Geometry check sheet. Reference: the model listing, model coordinates, mm. Round coordinates to 2 decimals unless told otherwise and drop trailing zeros. Order: outer loops, then holes, each group sorted by start corner. A loop starts at its lowest first (then second) coordinate and runs counter-clockwise, first axis right, second up.
(1) Cross-section at C-C on y = 1.75. Enter the section's corners in (x, z).
(2) Thickness scan on L1, parallel to X at y = 6.75, z = -0.25; L2, parallel to Z at x = -180, y = 6.25; L3, parallel to X at y = 6.5, z = -1. Record the ranges inside material, lowest first.
(3) Cross-section at A-A on z = 0. Enter the section's corners in (x, y).
(4) Gauge pin test, flat end, axial feed: P1, Ø1.5, axis at y = 3, z = -5.5, coming from the +X side. Record the tip position at first contact, or that the pin passes through.
(5) Cross-section at B-B on x = -160. Enter the section's corners in (y, z).
from build123d import *

# Parameters (mm, degrees)
BOSS_EXTRUDE1_DEPTH = 7.5
SKETCH2_R           = 2
CUT_EXTRUDE1_DEPTH  = 191.360841561
SKETCH3_R           = 5
CUT_EXTRUDE2_DEPTH  = 191.360841561


with BuildPart() as part:
    # Sketch1 → Boss-Extrude1 (new body)
    with BuildSketch(Plane(origin=(0, 0, 0), x_dir=(1, 0, 0), z_dir=(0, 1, 0))):
        with BuildLine():
            Line((0, 9), (-190, 9))
            Line((-190, 9), (-190, -9))
            Line((-190, -9), (0, -9))
            ThreePointArc((0, -9), (9, 0), (0, 9))
        make_face()
    extrude(amount=BOSS_EXTRUDE1_DEPTH)

    # Sketch2 → Cut-Extrude1 (cut, through all)
    with BuildSketch(Plane(origin=(0, 7.5, 0), x_dir=(1, 0, 0), z_dir=(0, 1, 0))):
        with Locations(Location((-180, 0, 0), (0, 0, 270))):
            Circle(SKETCH2_R)
        with Locations(Location((-160, 0, 0), (0, 0, 270))):
            Circle(SKETCH2_R)
    extrude(amount=-CUT_EXTRUDE1_DEPTH, mode=Mode.SUBTRACT)

    # Sketch3 → Cut-Extrude2 (cut, through all)
    with BuildSketch(Plane(origin=(0, 7.5, 0), x_dir=(1, 0, 0), z_dir=(0, 1, 0))):
        with Locations(Location((0, 0, 0), (0, 0, 270))):
            Circle(SKETCH3_R)
    extrude(amount=-CUT_EXTRUDE2_DEPTH, mode=Mode.SUBTRACT)


solid = part.part
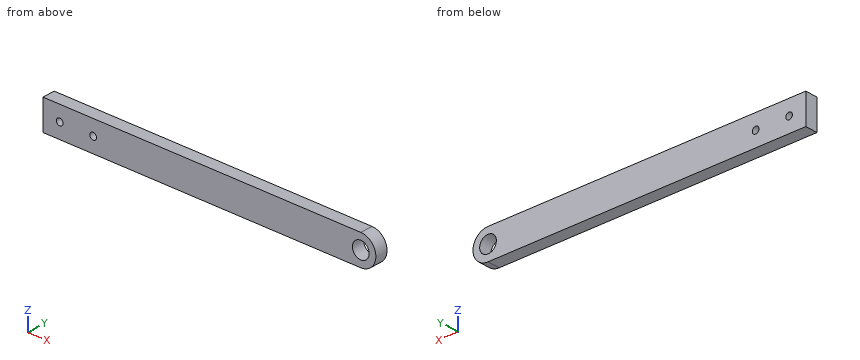
Found:
1. outline: (-190, -9) - (0, -9) arc R9 ccw to (0, 9) - (-190, 9) - close; hole circle Ø4 at (-180, 0); hole circle Ø4 at (-160, 0); hole circle Ø10 at (0, 0)
2. L1: x = -190 to -181.98, -178.02 to -161.98, -158.02 to -4.99, 4.99 to 9
2. L2: z = -9 to -2, 2 to 9
2. L3: x = -190 to -181.73, -178.27 to -161.73, -158.27 to -4.9, 4.9 to 8.94
3. outline: (-190, 0) - (-182, 0) - (-182, 7.5) - (-190, 7.5) - close; (-178, 0) - (-162, 0) - (-162, 7.5) - (-178, 7.5) - close; (-158, 0) - (-5, 0) - (-5, 7.5) - (-158, 7.5) - close; (5, 0) - (9, 0) - (9, 7.5) - (5, 7.5) - close
4. P1: stops at x = 7.64
5. outline: (0, -9) - (7.5, -9) - (7.5, -2) - (0, -2) - close; (0, 2) - (7.5, 2) - (7.5, 9) - (0, 9) - close
